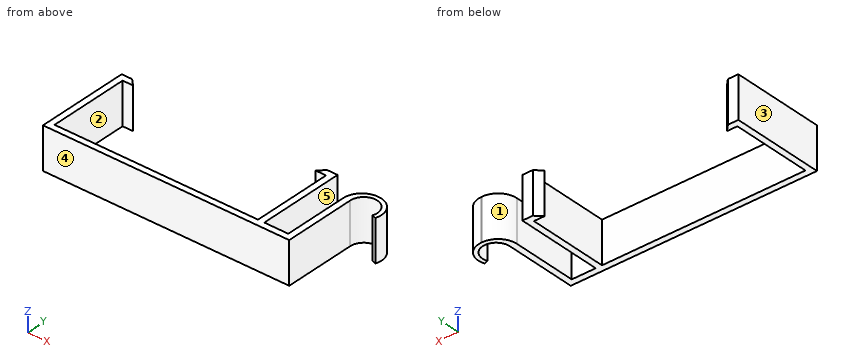
from build123d import *

# Parameters (mm, degrees)
F1_DEPTH = 20
F2_SIZE  = 2.99999
F3_R     = 9


# Not quite as in the source:
# - a fillet or chamfer is up to 0.001 mm smaller than in the source, because OpenCascade refuses the exact size


with BuildPart() as f1:
    # F0 (on Top) → F1 (new body)
    with BuildSketch(Plane.XY):
        with BuildLine():
            Line((0, 40), (0, 0))
            Line((0, 0), (-11.5, 0))
            Line((-11.5, 0), (-11.5, 41.5))
            Line((-11.5, 41.5), (-19.5, 41.5))
            Line((-19.5, 41.5), (-19.5, 38.5))
            Line((-19.5, 38.5), (-14.5, 38.5))
            Line((-14.5, 38.5), (-14.5, 0))
            Line((-14.5, 0), (-112, 0))
            Line((-112, 0), (-112, 38.5))
            Line((-112, 38.5), (-107, 38.5))
            Line((-107, 38.5), (-107, 41.5))
            Line((-107, 41.5), (-115, 41.5))
            Line((-115, 41.5), (-115, -3))
            Line((-115, -3), (3, -3))
            Line((3, -3), (3, 31.5))
            ThreePointArc((3, 31.5), (10.6287131548, 37.9012503946), (15.6080020351, 29.2768690684))
            Line((15.6080020351, 29.2768690684), (17.4873872767, 28.5928287817))
            ThreePointArc((17.4873872767, 28.5928287817), (16.4627923765, 36.375399709), (9.5, 40))
            Line((9.5, 40), (3, 40))
            Line((3, 40), (0, 40))
        make_face()
    extrude(amount=F1_DEPTH)

    # F2 (size 3 in the source; OpenCascade refuses exactly that, so slightly less here)
    f2_edges = [f1.edges().sort_by_distance(p)[0] for p in [
        (-107, 41.5, 10),
        (-19.5, 41.5, 10),
    ]]
    chamfer(f2_edges, length=F2_SIZE)

    # F3
    f3_edges = [f1.edges().sort_by_distance(p)[0] for p in [
        (0, 40, 10),
    ]]
    fillet(f3_edges, radius=F3_R)


solid = f1.part
Part model, mm, in its own coordinate system. Face numbers are marked on the shaded views. A direction names the side the tool comes from. Round coordinates to 2 decimals unless told otherwise and drop trailing zeros. Write each loop counter-clockwise with the first axis right and the second up, starting at its lowest first coordinate (ties: lowest second). Pieces come first, ordered by that corner, then holes. Notation, with made-up numbers: M 43.25,5.25 L 97.25,5.25 A15 ccw 97.25,15.25 Z; hole C 67.25,33.25 d4. An arc over 180 degrees is marked long. Return JSON: item names as keys, results as strings. Group by question number.
(1) Saw through at C-C on x = -41. Write the cut outline in (y, z).
(2) Drill centre lines: probe 1 along X at (y, z) = (15, 13.5); probe 2 along X at (y, z) = (31.5, 5.5); probe 3 along X at (y, z) = (33, 2). Where is each one in solid material? Low to high.
(3) Which spindle directions (+Z, -Z, +X, -X, +Y, -Y) get a long thin tool onto all of the face, cutting with end or side? Do the marked faces 1 and 2. Say none if no direction does.
(4) Pin check, flat tips, straight feed: pin 1 Ø6 at (x, z) = (-81, 10) entering from +Y; pin 2 Ø10 at (y, z) = (17.5, 9.5) entering from +X; pin 3 Ø12 at (x, y) = (-4.5, 22.5) entering from -Z; pin 4 Ø0.6 at (x, z) = (9, 6.5) entering from +Y. Stop position of each tip, or through.
(5) Saw through at A-A on y = 24. Write the cut outline in (x, z), then the cut area to 3 significant figures.
(6) Two-plate mould, pull along X, no slides. Class the marked faces 3, 4 and 5: +X half, -X half, draft (parallel to the pull), parting line (faces both ways), or undercut.
Returned:
{
 "1": {"outline": "M -3,0 L 0,0 L 0,20 L -3,20 Z"},
 "2": {"probe 1": "-115 to -112, -14.5 to -11.5, 0 to 3", "probe 2": "-115 to -112, -14.5 to -11.5, 0.01 to 3, 16 to 18", "probe 3": "-115 to -112, -14.5 to -11.5, 0.23 to 3.18, 15.82 to 17.87"},
 "3": {"face 1": "+Z, -Z, +Y", "face 2": "+Z, -Z"},
 "4": {"pin 1": "y = 0", "pin 2": "x = 3", "pin 3": "z = 0", "pin 4": "y = 40"},
 "5": {"outline": "M -115,0 L -112,0 L -112,20 L -115,20 Z; M -14.5,0 L -11.5,0 L -11.5,20 L -14.5,20 Z; M 0,0 L 3,0 L 3,20 L 0,20 Z", "area": "180 mm²"},
 "6": {"face 3": "-X half", "face 4": "draft", "face 5": "undercut"}
}
